The model under review builds one solid part; all positions refer to its coordinate system, in mm. Face numbers are marked on the shaded views. Round coordinates to 2 decimals unless told otherwise and drop trailing zeros. Loops run counter-clockwise (first coordinate to the right, second up) from the corner with the lowest first, then second, coordinate; pieces in that order, holes last. Notation, with made-up numbers: M -1.75,-24.5 L 41.25,-24.5 A23 ccw 41.25,-16.5 Z; hole C -32,54.5 d1. An arc over 180 degrees is marked long. Answer as a JSON object with one key per item and string values. Group by question number.
Item 1: Consider section A-A (y = -0.5). Give the boundary of the cut face in (x, z), and give its area (3 significant figures).
Item 2: Insertion check: P1, Ø5, axis at x = 1.47, y = -2.18, coming from the -Z side. The pin has a flat end and moves straight along its axis. Give the tip position at first contact, or say it passes through.
Item 3: Consider section C-C (z = 3). Give the boundary of the cut face in (x, y), and give its area (3 significant figures).
Item 4: Consider section B-B (x = 4). Give the boundary of the cut face in (y, z), and give its area (3 significant figures).
Item 5: The part is to be moulded in two halves that separate along Y. For the marked faces 1, 2, 3 and 4, say which applies: +Y half, -Y half, draft (parallel to the pull), parting line (faces both ways), or undercut.
Item 6: Consider section D-D (y = 3.25). Give the boundary of the cut face in (x, z), and give its area (3 significant figures).
Item 7: To check wall thickness, follow line 1 (X direction, y = -2.25, z = 1); line 2 (X direction, y = -2.25, z = 6.25); line 3 (X direction, y = 3.5, z = 5). State the ranges of each line that lie inside material, in increasing order.
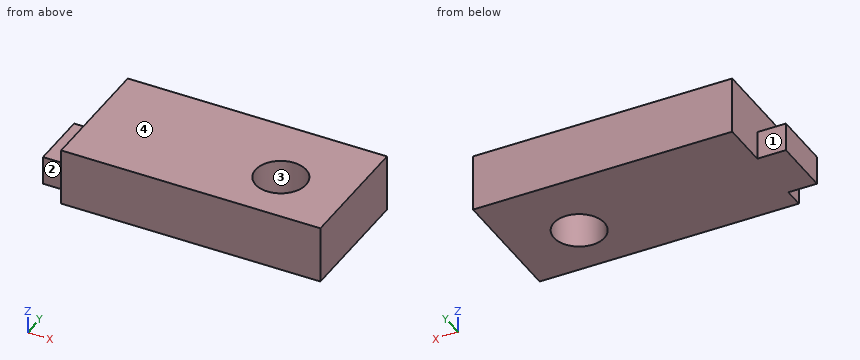
Autodesk Inventor part; units mm, degrees
ref_plane "YZ Plane" through (0, 0, 0) normal (1, 0, 0) x (0, 1, 0)
ref_plane "XZ Plane" through (0, 0, 0) normal (0, 1, 0) x (-1, 0, 0)
ref_plane "XY Plane" through (0, 0, 0) normal (0, 0, 1) x (1, 0, 0)
sketch "Sketch1" plane through (0, 0, 0) normal (0, 0, 1) x (1, 0, 0)
  line L0 (-21.2538, 6.4099) -> (9.5462, 6.4099)
  line L1 (9.5462, 6.4099) -> (9.5462, -8.5901)
  line L2 (9.5462, -8.5901) -> (-21.2538, -8.5901)
  line L3 (-21.2538, -8.5901) -> (-21.2538, 6.4099)
  line L4 (1.0462, -38.9134) -> (26.8462, -38.9134)
  line L5 (-4.9538, -50.9134) -> (0.0462, -50.9134)
  point P0 (0, 0)
  dimension "d0" = 30.8
  dimension "d1" = 15
  dimension "d8" = 25.8
  dimension "d9" = 5
extrude "Extrusion1" add sketch "Sketch1" along normal blind 6.8
sketch "Sketch2" plane through (0, 0, 6.8) normal (0, 0, 1) x (1, 0, 0)
  circle A0 centre (1.4656, -2.1794) radius 3
  circle A1 centre (1.4656, -2.1794) radius 3
  point P0 (0, 0)
extrude "Extrusion2" cut sketch "Sketch2" against normal blind 14
sketch "Sketch3" plane through (0, 0, 0) normal (0, 0, -1) x (-1, 0, 0)
  line L0 (5.4538, -4.4054) -> (8.8538, -4.4054)
  line L1 (5.4538, 2.5946) -> (8.8538, 2.5946)
  line L2 (8.8538, 84.2919) -> (8.8538, -65.7081)
  line L3 (5.4538, -4.4054) -> (8.8538, -4.4054)
  line L4 (8.8538, -4.4054) -> (8.8538, 2.5946)
  line L5 (8.8538, 2.5946) -> (5.4538, 2.5946)
  line L6 (5.4538, 2.5946) -> (5.4538, -4.4054)
  point P0 (0, 0)
extrude "Extrusion3" add sketch "Sketch3" against normal blind 3.4
sketch "Sketch4" plane through (-21.2538, -8.5901, 0) normal (-1, 0, 0) x (0, 0, 1)
  line L0 (3.4, 2.3591) -> (0, 2.3591)
  line L1 (3.4, 9.3591) -> (3.4, 2.3591)
  line L2 (3.4, 2.3591) -> (0, 2.3591)
  line L3 (0, 2.3591) -> (0, 9.3591)
  line L4 (0, 9.3591) -> (3.4, 9.3591)
  line L5 (3.4, 9.3591) -> (3.4, 2.3591)
  point P0 (0, 8.5901)
extrude "Extrusion4" add sketch "Sketch4" along normal blind 3.4
equation "\"d0\" = d8 + d9"
properties part number "Fixer"
Geometry results:
{
 "1": {"outline": "M -24.65,0 L -1.02,0 L -1.02,6.8 L -21.25,6.8 L -21.25,3.4 L -24.65,3.4 Z; M 3.95,0 L 9.55,0 L 9.55,6.8 L 3.95,6.8 Z", "area": "187 mm^2"},
 "2": {"P1": "passes through"},
 "3": {"outline": "M -24.65,-6.23 L -21.25,-6.23 L -21.25,-8.59 L 9.55,-8.59 L 9.55,6.41 L -21.25,6.41 L -21.25,0.77 L -24.65,0.77 Z; hole C 1.47,-2.18 d6", "area": "458 mm^2"},
 "4": {"outline": "M -8.59,0 L -3.78,0 L -3.78,6.8 L -8.59,6.8 Z; M -0.57,0 L 6.41,0 L 6.41,6.8 L -0.57,6.8 Z", "area": "80.2 mm^2"},
 "5": {"face 1": "+Y half", "face 2": "-Y half", "face 3": "undercut", "face 4": "draft"},
 "6": {"outline": "M -21.25,0 L 9.55,0 L 9.55,6.8 L -21.25,6.8 Z", "area": "209 mm^2"},
 "7": {"line 1": "x = -24.65 to -1.53, 4.46 to 9.55", "line 2": "x = -21.25 to -1.53, 4.46 to 9.55", "line 3": "x = -21.25 to 9.55"}
}
